Source: CAD feature listing. Evaluate the final solid. Frame: model axes, mm. Face numbers are marked on the shaded views. A direction names the side the tool comes from. Coordinates: 2 decimals unless noted, no trailing zeros. Order: outer loops, then holes, each group sorted by start corner. A loop starts at its lowest first (then second) coordinate and runs counter-clockwise, first axis right, second up.
```python
from build123d import *

# Parameters (mm, degrees)
SKETCH1_W           = 473
SKETCH1_H           = 217
BOSS_EXTRUDE1_DEPTH = 85
SKETCH2_W           = 280
SKETCH2_H           = 44
CUT_EXTRUDE1_DEPTH  = 15
SKETCH3_W           = 443
SKETCH3_H           = 187
CUT_EXTRUDE2_DEPTH  = 70
FILLET1_R           = 9
SKETCH4_W           = 90
SKETCH4_H           = 30
BOSS_EXTRUDE2_DEPTH = 8
SKETCH5_R           = 3
CUT_EXTRUDE3_DEPTH  = 15
SKETCH6_R           = 3
CUT_EXTRUDE4_DEPTH  = 15


with BuildPart() as part:
    # Sketch1 → Boss-Extrude1 (new body)
    with BuildSketch(Plane(origin=(0, 0, 0), x_dir=(1, 0, 0), z_dir=(0, 1, 0))):
        Rectangle(SKETCH1_W, SKETCH1_H)
    extrude(amount=BOSS_EXTRUDE1_DEPTH)

    # Sketch2 → Cut-Extrude1 (cut)
    with BuildSketch(Plane(origin=(0, 85, 0), x_dir=(1, 0, 0), z_dir=(0, 1, 0))):
        with Locations((-81.5, 56.5)):
            Rectangle(SKETCH2_W, SKETCH2_H)
    extrude(amount=-CUT_EXTRUDE1_DEPTH, mode=Mode.SUBTRACT)

    # Sketch3 → Cut-Extrude2 (cut)
    with BuildSketch(Plane.XZ):
        Rectangle(SKETCH3_W, SKETCH3_H)
    extrude(amount=-CUT_EXTRUDE2_DEPTH, mode=Mode.SUBTRACT)

    # Fillet1
    fillet1_edges = [part.edges().sort_by_distance(p)[0] for p in [
        (-221.5, 77.5, -34.5),
        (-221.5, 77.5, -78.5),
        (58.5, 77.5, -78.5),
        (58.5, 77.5, -34.5),
    ]]
    fillet(fillet1_edges, radius=FILLET1_R)

    # Sketch4 → Boss-Extrude2 (add)
    with BuildSketch(Plane(origin=(0, 85, 0), x_dir=(1, 0, 0), z_dir=(0, 1, 0))):
        with Locations((-87.81, 93.5)):
            Rectangle(SKETCH4_W, SKETCH4_H)
    extrude(amount=BOSS_EXTRUDE2_DEPTH)

    # Sketch5 → Cut-Extrude3 (cut)
    with BuildSketch(Plane(origin=(0, 93, 0), x_dir=(1, 0, 0), z_dir=(0, 1, 0))):
        with Locations(Location((-112.31, 93.5, 0), (0, 0, 270))):
            Circle(SKETCH5_R)
        with Locations(Location((-67.31, 93.5, 0), (0, 0, 270))):
            Circle(SKETCH5_R)
    extrude(amount=-CUT_EXTRUDE3_DEPTH, mode=Mode.SUBTRACT)

    # Sketch6 → Cut-Extrude4 (cut)
    with BuildSketch(Plane(origin=(0, 85, 0), x_dir=(1, 0, 0), z_dir=(0, 1, 0))):
        with Locations(Location((-127.5, -82.5, 0), (0, 0, 270))):
            Circle(SKETCH6_R)
        with Locations(Location((-127.5, -14.5, 0), (0, 0, 270))):
            Circle(SKETCH6_R)
        with Locations(Location((38.5, -14.5, 0), (0, 0, 270))):
            Circle(SKETCH6_R)
        with Locations(Location((204.5, -14.5, 0), (0, 0, 270))):
            Circle(SKETCH6_R)
        with Locations(Location((204.5, -82.5, 0), (0, 0, 270))):
            Circle(SKETCH6_R)
        with Locations(Location((38.5, -82.5, 0), (0, 0, 270))):
            Circle(SKETCH6_R)
    extrude(amount=-CUT_EXTRUDE4_DEPTH, mode=Mode.SUBTRACT)


solid = part.part
```
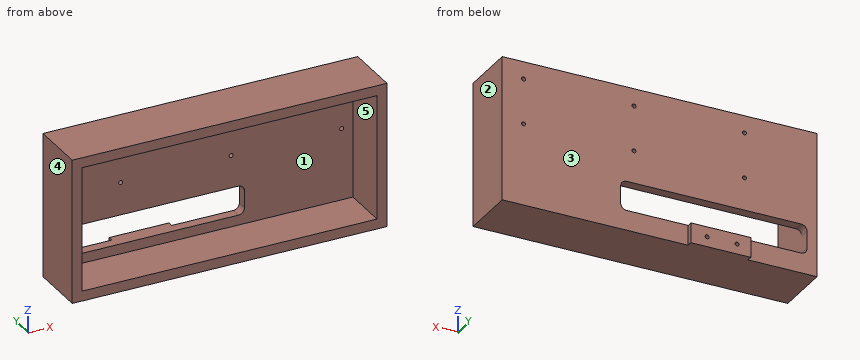
Q1. Section query A-A on z = -52. Output: boundary loops of the cut face in (x, y).
Solutions:
outline: (-236.5, 0) - (-221.5, 0) - (-221.5, 85) - (-236.5, 85) - close; (58.5, 70) - (221.5, 70) - (221.5, 0) - (236.5, 0) - (236.5, 85) - (58.5, 85) - close
Q2. Section query D-D on x = 175.5. Output: boundary loops of the cut face in (y, z).
Solutions:
outline: (0, -108.5) - (85, -108.5) - (85, 108.5) - (0, 108.5) - (0, 93.5) - (70, 93.5) - (70, -93.5) - (0, -93.5) - close
Q3. Pin query (flat end, axial travel): P1, Ø4, axis at y = 88, z = -94.5, coming from the +X side; P2, Ø8, axis at x = 38.5, z = 14.5, coming from the +Y side; P3, Ø5.5, axis at x = 204.5, z = 14.5, coming from the +Y side; P4, Ø1.5, axis at x = -4.5, z = 21.5, coming from the -Y side. Return the tip coordinate at first contact, or that it passes through.
Solutions:
P1: stops at x = -42.81
P2: stops at y = 85
P3: passes through
P4: stops at y = 70
Q4. Section query C-C on y = 15. Output: boundary loops of the cut face in (x, z).
Solutions:
outline: (-236.5, -108.5) - (236.5, -108.5) - (236.5, 108.5) - (-236.5, 108.5) - close; hole (-221.5, -93.5) - (221.5, -93.5) - (221.5, 93.5) - (-221.5, 93.5) - close
Q5. Pull-direction query (X, two-part tool) for the marked faces 3, 4 and 5; classes: pulls with the +X half, pulls with the -X half, needs draft (parallel to the pull), parting line crosses it, or undercut.
Solutions:
face 3: needs draft
face 4: pulls with the -X half
face 5: undercut
Q6. Material intervals for line 1 along X through (y, z) = (80.5, 14.5); line 2 along Z through (x, y) = (-127, 77); line 3 along Z through (x, y) = (204.5, 75), sorted ascending.
Solutions:
line 1: x = -236.5 to -130.5, -124.5 to 35.5, 41.5 to 201.5, 207.5 to 236.5
line 2: z = -108.5 to -78.5, -34.5 to 11.54, 17.46 to 79.54, 85.46 to 108.5
line 3: z = -108.5 to 11.5, 17.5 to 79.5, 85.5 to 108.5
Q7. Section query B-B on x = -20. Output: boundary loops of the cut face in (y, z).
Solutions:
outline: (0, -108.5) - (85, -108.5) - (85, -78.5) - (70, -78.5) - (70, -93.5) - (0, -93.5) - close; (0, 93.5) - (70, 93.5) - (70, -34.5) - (85, -34.5) - (85, 108.5) - (0, 108.5) - close
Q8. Set-up query: the marked faces 1 and 2. Return all of +Z, -Z, +X, -X, +Y, -Y with unobstructed straight access to the full face (end or side cutting, diameter ignored); none if empty.
Solutions:
face 1: -Y
face 2: +Z, -Z, +X, +Y, -Y
